Geometry check sheet. Reference: the model listing, model coordinates, mm. A direction names the side the tool comes from. Round coordinates to 2 decimals unless told otherwise and drop trailing zeros. Order: outer loops, then holes, each group sorted by start corner. A loop starts at its lowest first (then second) coordinate and runs counter-clockwise, first axis right, second up. Notation, with made-up numbers: (-15, 44) - (22, 44) arc R21 cw to (22, 69) - close; hole circle Ø2 at (29.25, -34.75). An arc over 180 degrees is marked (long way). Use a Markdown table: item, result. Add a question column.
(1) Gauge pin test, flat ends, axial feed: P1, Ø1.5, axis at y = 35, z = 13, coming from the -X side; P2, Ø3, axis at x = 3.5, y = 19.5, coming from the +Z side; P3, Ø1.5, axis at x = 3.5, y = 11, coming from the -Z side; P4, Ø8, axis at x = 15, y = 34.5, coming from the +Z side. Record the tip position at first contact, or that the pin passes through.
(2) Mould release check, pull along X, two halves, no side actions. Record for faces 4 (the face through (19.43, 0.6, 1.01)), 5 (the face through (-9.5, 7, 1)), 6 (the face through (0, 38, -1)): released by +X, released by -X, zero draft, split by the parting line, or undercut.
(3) Section check D-D on z = 4.75. Record the boundary of the cut face in (x, y).
(4) Section check B-B on x = 0. Record the boundary of the cut face in (y, z).
(5) Section check C-C on y = 18. Record the boundary of the cut face in (x, z).
(6) Section check A-A on x = 12.75. Record the boundary of the cut face in (y, z).
(7) Thickness scan on line 1 along Z through (x, y) = (-5.5, 23.5); line 2 along X through (y, z) = (35.5, 12.5); line 3 along Y through (x, z) = (4, 9.5). Record the ranges inside material, lowest first. Write a range as [from, to].
(8) Access from +Z, -Z, +X, -X, +Y, -Y to the whole of each face (thin tool, end or side, straight path). Record for faces 1 (the face through (-19.43, 0.6, 1.01)), 2 (the face through (-1.19, 38.59, -0.25)), 3 (the face through (12.82, 11.75, 0.99)).
```python
from build123d import *

# Parameters (mm, degrees)
PAD_DEPTH    = 2
SKETCH001_R  = 6
PAD001_DEPTH = 15
SKETCH002_R  = 1.5
PAD002_DEPTH = 1
FILLET_R     = 2
FILLET001_R  = 0.6
CHAMFER_SIZE = 0.5


with BuildPart() as part:
    # Sketch → Pad (new body)
    with BuildSketch(Plane.XY):
        with BuildLine():
            Line((-20, 0), (20, 0))
            Line((20, 0), (20, 20))
            Line((20, 20), (4.882401, 41.164639))
            ThreePointArc((4.882401, 41.164639), (0, 43.67721), (-4.882401, 41.164639))
            Line((-4.882401, 41.164639), (-20, 20))
            Line((-20, 20), (-20, 0))
        make_face()
        with BuildLine():
            ThreePointArc((16, 8.5), (12.75, 11.75), (9.5, 8.5))
            Line((9.5, 8.5), (9.5, 5))
            ThreePointArc((9.5, 5), (12.75, 1.75), (16, 5))
            Line((16, 8.5), (16, 5))
        make_face(mode=Mode.SUBTRACT)
        with BuildLine():
            ThreePointArc((-9.5, 8.5), (-12.75, 11.75), (-16, 8.5))
            Line((-16, 8.5), (-16, 5))
            ThreePointArc((-16, 5), (-12.75, 1.75), (-9.5, 5))
            Line((-9.5, 8.5), (-9.5, 5))
        make_face(mode=Mode.SUBTRACT)
    extrude(amount=PAD_DEPTH)

    # Sketch001 (on Face16 of Pad) → Pad001 (join)
    with BuildSketch(Plane.XY.offset(2)):
        with Locations((0, 37.67721)):
            Circle(SKETCH001_R)
    extrude(amount=PAD001_DEPTH)

    # Sketch002 (on Face4 of Pad001) → Pad002 (join)
    with BuildSketch(Plane(origin=(0, 0, 0), x_dir=(1, 0, 0), z_dir=(0, 0, -1))):
        with Locations((0, -37.67721)):
            Circle(SKETCH002_R)
    extrude(amount=PAD002_DEPTH)

    # Fillet
    fillet_edges = [part.edges().sort_by_distance(p)[0] for p in [
        (20, 0, 1),
        (-20, 0, 1),
        (-20, 20, 1),
        (20, 20, 1),
    ]]
    fillet(fillet_edges, radius=FILLET_R)

    # Fillet001
    fillet001_edges = [part.edges().sort_by_distance(p)[0] for p in [
        (-6, 37.67721, 17),
    ]]
    fillet(fillet001_edges, radius=FILLET001_R)

    # Chamfer
    chamfer_edges = [part.edges().sort_by_distance(p)[0] for p in [
        (-1.5, 37.67721, -1),
    ]]
    chamfer(chamfer_edges, length=CHAMFER_SIZE)


solid = part.part
```
Check sheet entries:
| question | item | result |
|---|---|---|
| 1 | P1 | stops at x = -5.68 |
| 1 | P2 | stops at z = 2 |
| 1 | P3 | stops at z = 0 |
| 1 | P4 | passes through |
| 2 | face 4 | released by +X |
| 2 | face 5 | undercut |
| 2 | face 6 | zero draft |
| 3 | outline | circle Ø12 at (0, 37.68) |
| 4 | outline | (0, 0) - (36.18, 0) - (36.18, -0.5) - (36.68, -1) - (38.68, -1) - (39.18, -0.5) - (39.18, 0) - (43.68, 0) - (43.68, 16.4) arc R0.6 ccw to (43.08, 17) - (32.28, 17) arc R0.6 ccw to (31.68, 16.4) - (31.68, 2) - (0, 2) - close |
| 5 | outline | (-20, 0) - (20, 0) - (20, 2) - (-20, 2) - close |
| 6 | outline | (0, 0) - (1.75, 0) - (1.75, 2) - (0, 2) - close; (11.75, 0) - (30.15, 0) - (30.15, 2) - (11.75, 2) - close |
| 7 | line 1 | z = [0, 2] |
| 7 | line 2 | x = [-5.59, 5.59] |
| 7 | line 3 | y = [33.21, 42.15] |
| 8 | face 1 | +Z, -Z, -X, -Y |
| 8 | face 2 | -Z |
| 8 | face 3 | +Z, -Z |
